Model file for the job. Use its own axes, mm. Face numbers are marked on the shaded views. Round coordinates to 2 decimals unless told otherwise and drop trailing zeros. Order: outer loops, then holes, each group sorted by start corner. A loop starts at its lowest first (then second) coordinate and runs counter-clockwise, first axis right, second up. Notation, with made-up numbers: (85.5, 88) - (95.5, 88) arc R28 cw to (95.5, 111) - close; hole circle Ø6 at (32.25, -16). An arc over 180 degrees is marked (long way). Write item = value, one per line.
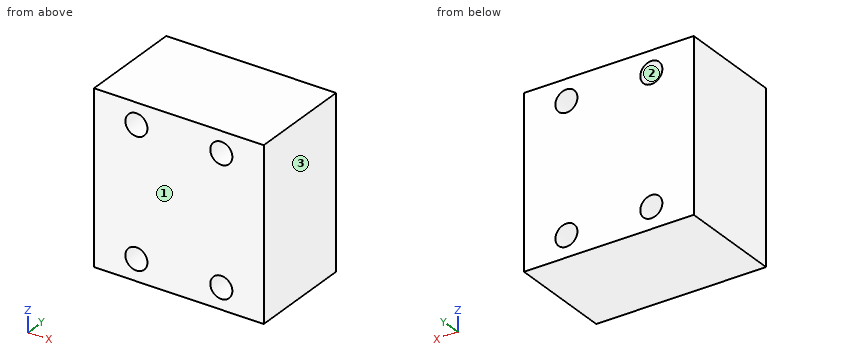
```python
from build123d import *

# Parameters (mm, degrees)
EXTRUDE_1_DEPTH      = 12.5
EXTRUDE_1_DEPTH_BACK = 12.5
SKETCH_1_W           = 40
SKETCH_1_H           = 40
SKETCH_2_R           = 2.6
CUT_EXTRUDE_3_DEPTH  = 38.749172176


with BuildPart() as part:
    # Sketch 1 → Extrude 1 (new, two sides: drawn at the far end of the back side and taken through both)
    with BuildSketch(Plane(origin=(0, 0, 0), x_dir=(1, 0, 0), z_dir=(0, 1, 0)).offset(-EXTRUDE_1_DEPTH_BACK)):
        Rectangle(SKETCH_1_W, SKETCH_1_H)
    extrude(amount=EXTRUDE_1_DEPTH + EXTRUDE_1_DEPTH_BACK)

    # Sketch 2 → Cut-Extrude 3 (cut, through all)
    with BuildSketch(Plane(origin=(0, 12.5, 0), x_dir=(1, 0, 0), z_dir=(0, 1, 0))):
        with Locations(Location((-10, 15, 0), (0, 0, 270))):
            Circle(SKETCH_2_R)
        with Locations(Location((10, 15, 0), (0, 0, 270))):
            Circle(SKETCH_2_R)
        with Locations(Location((-10, -15, 0), (0, 0, 270))):
            Circle(SKETCH_2_R)
        with Locations(Location((10, -15, 0), (0, 0, 270))):
            Circle(SKETCH_2_R)
    extrude(amount=-CUT_EXTRUDE_3_DEPTH, mode=Mode.SUBTRACT)


solid = part.part
```
1) Cut at C-C (y = -6.25). Write the cut outline in (x, z).
Conclusion:
outline = (-20, -20) - (20, -20) - (20, 20) - (-20, 20) - close; hole circle Ø5.2 at (-10, -15); hole circle Ø5.2 at (-10, 15); hole circle Ø5.2 at (10, -15); hole circle Ø5.2 at (10, 15)
2) Cut at B-B (z = 15). Write the cut outline in (x, y), and give its area (3 significant figures).
Conclusion:
outline = (-20, -12.5) - (-12.6, -12.5) - (-12.6, 12.5) - (-20, 12.5) - close; (-7.4, -12.5) - (7.4, -12.5) - (7.4, 12.5) - (-7.4, 12.5) - close; (12.6, -12.5) - (20, -12.5) - (20, 12.5) - (12.6, 12.5) - close
area = 740 mm^2
3) Wall check: line 1 along X through (y, z) = (-1.5, 15); line 2 along X through (y, z) = (-2.25, -13); line 3 along Z through (x, y) = (-10.5, 0). Give the ranges that are in metal, low to high.
Conclusion:
line_1 = -20 to -12.6, -7.4 to 7.4, 12.6 to 20
line_2 = -20 to -11.66, -8.34 to 8.34, 11.66 to 20
line_3 = -20 to -17.55, -12.45 to 12.45, 17.55 to 20
4) Flat gauge pin, fed straight in: pin 1 Ø7 at (x, z) = (-10, -15) entering from +Y. Where does the tip first touch, or does it go through?
Conclusion:
pin_1 = 12.5
5) Cut at A-A (x = -10). Write the cut outline in (y, z).
Conclusion:
outline = (-12.5, -20) - (12.5, -20) - (12.5, -17.6) - (-12.5, -17.6) - close; (-12.5, -12.4) - (12.5, -12.4) - (12.5, 12.4) - (-12.5, 12.4) - close; (-12.5, 17.6) - (12.5, 17.6) - (12.5, 20) - (-12.5, 20) - close
6) Mould opens along X. For the marked faces 1, 2 and 3 say: +X half, -X half, draft (parallel to the pull), parting line (faces both ways), or undercut.
Conclusion:
face_1 = draft
face_2 = undercut
face_3 = +X half
